```python
from build123d import *

# Parameters (mm, degrees)
BASEHEAD_DEPTH = 6.4
SKETCH5_R      = 5
BASEBODY_DEPTH = 110
CHAMFER1_SIZE  = 0.5


with BuildPart() as part:
    # Sketch2 → BaseHead (new body)
    with BuildSketch(Plane(origin=(0, 0, 0), x_dir=(0, 0, -1), z_dir=(1, 0, 0))):
        Polygon((0, -9.237604307), (8, -4.618802154), (8, 4.618802154), (0, 9.237604307), (-8, 4.618802154), (-8, -4.618802154), align=None)
    extrude(amount=BASEHEAD_DEPTH)

    # Sketch3 → BearingFace (revolve, cut)
    with BuildSketch(Plane.XY, mode=Mode.PRIVATE) as bearingface_sk:
        Polygon((6.4, 9.237604307), (6.4, 7.235), (5.8, 7.835), (5.8, 9.237604307), align=None)
    revolve(bearingface_sk.sketch.rotate(Axis((-0.957090588, 0, 0), (1, 0, 0)), 90), axis=Axis((-0.957090588, 0, 0), (1, 0, 0)), mode=Mode.SUBTRACT)

    # Sketch4 → HeadChamfer (revolve, cut)
    with BuildSketch(Plane.XY):
        Polygon((0, 9.237604307), (0.45045113, 9.237604307), (0, 8), align=None)
    revolve(axis=Axis((-0.493528746, 0, 0), (1, 0, 0)), mode=Mode.SUBTRACT)

    # Sketch5 → BaseBody (add)
    with BuildSketch(Plane(origin=(6.4, 0, 0), x_dir=(0, 0, -1), z_dir=(1, 0, 0))):
        with Locations(Location((0, 0, 0), (0, 0, 180))):
            Circle(SKETCH5_R)
    extrude(amount=BASEBODY_DEPTH)

    # Chamfer1
    chamfer1_edges = [part.edges().sort_by_distance(p)[0] for p in [
        (116.4, 0, -5),
    ]]
    chamfer(chamfer1_edges, length=CHAMFER1_SIZE)


solid = part.part
```
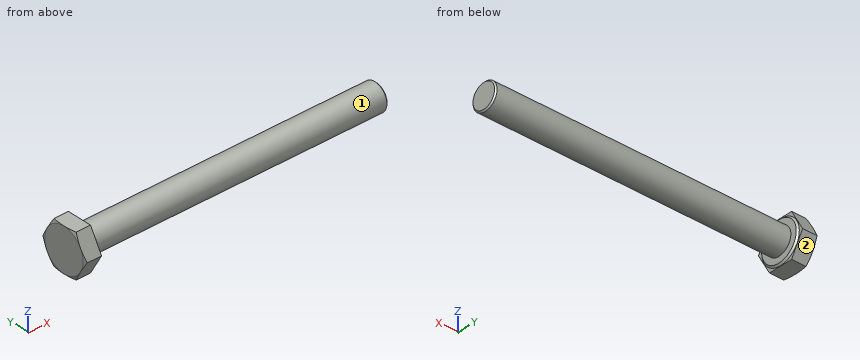
The listing builds one solid part. Answer for the finished solid, in the listing's coordinates (mm). Face numbers are marked on the shaded views. A direction names the side the tool comes from. Give positions to 0.01 mm unless a question says otherwise; leave off trailing zeros. Write each loop counter-clockwise with the first axis right and the second up, starting at its lowest first coordinate (ties: lowest second). Pieces come first, ordered by that corner, then holes. Notation, with made-up numbers: (57.25, -11.5) -> (64.25, -11.5) arc R24 cw to (64.25, 12.5) -> close; hole circle Ø3 at (9.25, -6). An arc over 180 degrees is marked (long way). Write item = value, one per line. Start each with the question number.
1) Each of these flat-tipped pins is pushed along its axis until it touches: pin 1 (2 mm diameter, centred on x = 40.5, y = -1, fed in from -Z); pin 2 (2 mm diameter, centred on x = 56.5, y = -3.5, fed in from +Z); pin 3 (1 mm diameter, centred on y = 5, z = 0.5, fed in from +X). Where does it stop, or does it pass through?
2) Which of the six approach directions +Z, -Z, +X, -X, +Y, -Y give full straight-line access (tool end or side, diameter ignored) to the marked faces 1 and 2?
3) Straight lines are drawn through the part: line 1 along X through (y, z) = (2.5, -4.5); line 2 along Y through (x, z) = (67.5, -0.25); line 3 along Z through (x, y) = (27, 2.25). For each, find the intervals that lie inside material, in ascending order.
4) The part is cut by section A-A, the plane x = 25. Determine the outline of the cut face in (y, z).
Solutions:
q1.pin_1 = -5
q1.pin_2 = 4.33
q1.pin_3 = 116.38
q2.face_1 = +X
q2.face_2 = -Z, +X, -X, +Y
q3.line_1 = 0 to 6.4
q3.line_2 = -4.99 to 4.99
q3.line_3 = -4.47 to 4.47
q4.outline = circle Ø10 at (0, 0)
